Autodesk Inventor part; units mm, degrees
sketch "Sketch1" plane through (0, 0, 0) normal (1, 0, 0) x (0, 1, 0)
  line L0 (50, 25) -> (-50, 25)
  line L1 (-50, 25) -> (-50, -25)
  line L2 (-50, -25) -> (50, -25)
  line L3 (50, -25) -> (50, 25)
  line L4 (-70, 0) -> (70, 0)
  line L5 (0, 35) -> (0, -35)
  line L6 (-50, 25) -> (50, -25)
  line L7 (-36.7082, 15) -> (30, -18.3541)
  line L8 (-36.7082, 15) -> (-50, 15)
  line L9 (30, -25) -> (30, -18.3541)
  line L10 (30, -21.8) -> (33, -21.8)
  line L11 (33, -21.8) -> (33, -23.4)
  line L12 (33, -23.4) -> (30, -23.4)
  line L13 (30, -23.4) -> (30, -21.8)
  line L14 (33, -21.8) -> (31.4, -21.8)
  line L15 (31.4, -21.8) -> (31.4, -20.2)
  line L16 (31.4, -20.2) -> (33, -20.2)
  line L17 (33, -20.2) -> (33, -21.8)
  point P0 (0, 0)
  point P1 (50, 0)
  point P2 (0, 25)
  point P3 (43.2918, -25)
  point P4 (-50, 21.6459)
  dimension "d0" = 50
  dimension "d1" = 100
  dimension "d2" = 3
  dimension "d5" = 10
  dimension "d6" = 20
  dimension "d95" = 3
  dimension "d96" = 1.6
  dimension "d97" = 1.6
  dimension "d98" = 1.6
  dimension "d99" = 1.6
extrude "Extrusion1" add sketch "Sketch1" along normal mid plane 100 contours L6 L4 L7 L8 L1 | L5 L7 L4 | L6 L2 L9 L12 L11 L17 L16 L15 L10 L7 L5
sketch "Sketch4" plane through (50, 50, -25) normal (0, 0, -1) x (-1, 0, 0)
  circle A0 centre (5, -5) radius 1.5
  line L0 (0, -20) -> (0, 0)
  line L1 (100, 0) -> (0, 0)
  line L2 (5, -3.5) -> (5, -6.5)
  circle A1 centre (35, -5) radius 1.5
  line L3 (35, -3.5) -> (35, -6.5)
  circle A2 centre (65, -5) radius 1.5
  line L4 (65, -3.5) -> (65, -6.5)
  circle A3 centre (95, -5) radius 1.5
  line L5 (95, -3.5) -> (95, -6.5)
  point P0 (50, -50)
  point P1 (0, -100)
  dimension "d45" = 3
  dimension "d46" = 5
  dimension "d47" = 5
  dimension "d48" = 3
  dimension "d107" = 3
  dimension "d108" = 5
  dimension "d109" = 30
  dimension "d110" = 3
  dimension "d120" = 60
  dimension "d127" = 60
revolve "Revolution2" add sketch "Sketch4" angle 360 about axis through (45, 46.5, -25) along (0, -1, 0) picked at (4.5036, -4.9397) contours L2 A0
revolve "Revolution3" cut sketch "Sketch4" angle 360 about axis through (15, 46.5, -25) along (0, -1, 0) picked at (34.5036, -5.0603) contours L3 A1
revolve "Revolution4" add sketch "Sketch4" angle 360 about axis through (-15, 46.5, -25) along (0, -1, 0) picked at (64.2365, -5.2413) contours L4 A2
revolve "Revolution5" cut sketch "Sketch4" angle 360 about axis through (-45, 46.5, -25) along (0, -1, 0) picked at (94.1238, -4.716) contours L5 A3
sketch "Sketch5" plane through (-50, -50, 15) normal (0, -1, 0) x (1, 0, 0)
  circle A0 centre (5, 5) radius 2.5
  line L0 (0, 0) -> (0, 10)
  line L1 (0, 10) -> (100, 10)
  line L2 (50, 20) -> (50, -50)
  circle A1 centre (95, 5) radius 2.5
  line L3 (0, 5) -> (100, 5)
  line L4 (100, -40) -> (100, 10)
  point P0 (50, -15)
  dimension "d76" = 5
  dimension "d77" = 5
extrude "Extrusion3" add sketch "Sketch5" along normal blind 5 contours L3 A0 | A0 L3 | L3 A1 | A1 L3
properties part number "Roof_Large"
The model under review builds one solid part; all positions refer to its coordinate system, in mm. A direction names the side the tool comes from. Give positions to 0.01 mm unless a question says otherwise; leave off trailing zeros. Write each loop counter-clockwise with the first axis right and the second up, starting at its lowest first coordinate (ties: lowest second). Pieces come first, ordered by that corner, then holes. Notation, with made-up numbers: (41.25, -28) -> (94.25, -28) arc R22 ccw to (94.25, -14) -> close; hole circle Ø7 at (26.25, 18.25). An arc over 180 degrees is marked (long way). Answer in a Markdown table with one row per item.
1) Clearance check with flat-ended pins moving along their axes: P1, Ø4, axis at x = -18.5, y = -46.5, coming from the -Z side; P2, Ø1.5, axis at x = 14, y = 36.5, coming from the -Z side; P3, Ø2.5, axis at x = 9.5, y = 31.5, coming from the +Z side (3 decimals). State where each tip first meets the part, or that it passes through.
Worked answers:
| item | result |
|---|---|
| P1 | z = 15 |
| P2 | z = -25 |
| P3 | z = -15.125 |
2) For L1, parallel to Y at x = 17.5, z = -9.5; L2, parallel to Y at x = 11, z = -18; L3, parallel to Z at x = -8.5, y = -20, list the stretches that pass through material, from the lowest coordinate up. Write a range as [from, to].
Worked answers:
| item | result |
|---|---|
| L1 | [12.29, 19] |
| L2 | [29.29, 36] |
| L3 | [6.65, 10] |
3) Add section D-D on x = -45. State the section outline as (y, z) points.
Worked answers:
| item | result |
|---|---|
| outline | (-55, 17.5) -> (-50, 17.5) -> (-50, 15) -> (-36.71, 15) -> (30, -18.35) -> (30, -21.8) -> (31.4, -21.8) -> (31.4, -20.2) -> (33, -20.2) -> (33, -23.4) -> (30, -23.4) -> (30, -25) -> (43.5, -25) arc R1.5 cw to (46.5, -25) -> (50, -25) -> (-50, 25) -> (-50, 22.5) -> (-55, 22.5) -> close |
4) Add section A-A on x = 45. State the section outline as (y, z) points.
Worked answers:
| item | result |
|---|---|
| outline | (-55, 17.5) -> (-50, 17.5) -> (-50, 15) -> (-36.71, 15) -> (30, -18.35) -> (30, -21.8) -> (31.4, -21.8) -> (31.4, -20.2) -> (33, -20.2) -> (33, -23.4) -> (30, -23.4) -> (30, -25) -> (43.5, -25) arc R1.5 ccw to (46.5, -25) -> (50, -25) -> (-50, 25) -> (-50, 22.5) -> (-55, 22.5) -> close |
5) Tool access review of faces 5 (the cylindrical face through (47.385, -52.465, 19.249)), 6 (the flat face through (45, -55, 20)), 7 (the flat face through (-1, 30, -20)): name each direction out of +Z, -Z, +X, -X, +Y, -Y from which nothing blocks a thin tool from reaching the whole face with its end or side.
Worked answers:
| item | result |
|---|---|
| face 5 | -Y |
| face 6 | +Z, -Z, +X, -X, -Y |
| face 7 | -Z, +X, -X, -Y |
6) Add section B-B on z = 20. State the section outline as (x, y) points, plus the area to 3 significant figures.
Worked answers:
| item | result |
|---|---|
| outline | (-50, -50) -> (-47.5, -50) -> (-47.5, -55) -> (-42.5, -55) -> (-42.5, -50) -> (42.5, -50) -> (42.5, -55) -> (47.5, -55) -> (47.5, -50) -> (50, -50) -> (50, -40) -> (-50, -40) -> close |
| area | 1,050 mm² |
7) Mouldability with a two-part tool opening along Z and no side actions: class faces 1 (the flat face through (-1, 33, -22)), 2 (the flat face through (-0.7, -0.7, 0.35)), 3 (the cylindrical face through (-42.615, -52.465, 19.249)), 4 (the flat face through (-1, 32, -23.4)) as +Z half, -Z half, draft (parallel to the pull), parting line (faces both ways), or undercut.
Worked answers:
| item | result |
|---|---|
| face 1 | undercut |
| face 2 | +Z half |
| face 3 | parting line |
| face 4 | undercut |
8) Add section C-C on y = -38. State the section outline as (x, z) points, plus the area to 3 significant figures.
Worked answers:
| item | result |
|---|---|
| outline | (-50, 15) -> (50, 15) -> (50, 19) -> (-50, 19) -> close |
| area | 400 mm² |
